Read the model definition and answer for the solid it produces. Units are mm, in the model's axes. Face numbers are marked on the shaded views. Coordinates: 2 decimals unless noted, no trailing zeros. Write each loop counter-clockwise with the first axis right and the second up, starting at its lowest first coordinate (ties: lowest second). Pieces come first, ordered by that corner, then holes. Notation, with made-up numbers: (-3.75, 78) -> (12.25, 78) arc R24 ccw to (12.25, 98) -> close; hole circle Ø6 at (60.25, 6). An arc over 180 degrees is marked (long way). One line per item, written item: value. Start each with the question number.
1. Given P1, Ø4, axis at y = -2, z = 3, coming from the +X side; P2, Ø1.9, axis at x = 0, y = 1.5, coming from the +Z side; P3, Ø6, axis at x = -3.5, z = 8, coming from the -Y side, each flat-ended and moving along its own axis, determine where each tip first touches the part or whether it passes through.
2. Consider line 1 along Y through (x, z) = (0, 8) (3 decimals); line 2 along Y through (x, z) = (0, 1.2); line 3 along Z through (x, y) = (1.25, 1). Determine where each line is inside the solid, lowest interval first.
3. Find section C-C, the plane y = -1.25. Write down the section's boundary in (x, z), and give its area (3 significant figures).
4. For a pull along X with two mould halves and no side action, classify the marked faces 1, 2, 3 and 4 as pulls with the +X half, pulls with the -X half, needs draft (parallel to the pull), parting line crosses it, or undercut.
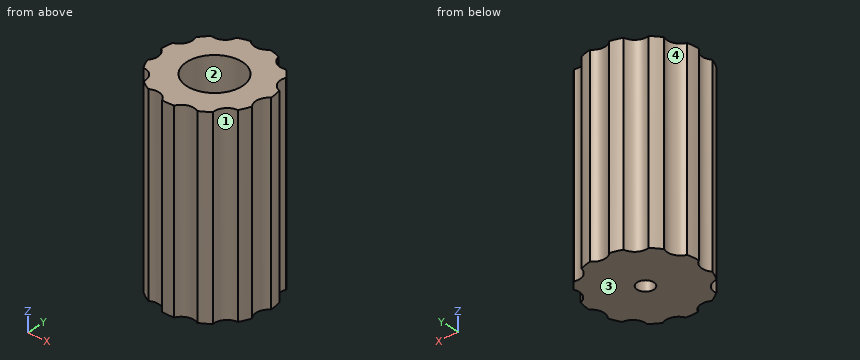
```python
from build123d import *

# Parameters (mm, degrees)
SKETCH1_R           = 6.35
BOSS_EXTRUDE1_DEPTH = 22
CUT_EXTRUDE1_DEPTH  = 23
CIRPATTERN1_COUNT   = 11
SKETCH3_R           = 3.175
CUT_EXTRUDE2_DEPTH  = 19
SKETCH4_R           = 0.9525
CUT_EXTRUDE3_DEPTH  = 4


with BuildPart() as part:
    # Sketch1 → Boss-Extrude1 (new body)
    with BuildSketch(Plane.XY):
        Circle(SKETCH1_R)
    extrude(amount=BOSS_EXTRUDE1_DEPTH)

    # Sketch2 → Cut-Extrude1 (cut, through all)
    with BuildSketch(Plane.XY.offset(22)):
        with BuildLine():
            ThreePointArc((-1.111662599, 6.251936201), (0, 5.75547169), (1.111662599, 6.251936201))
            ThreePointArc((1.111662599, 6.251936201), (0, 6.35), (-1.111662599, 6.251936201))
        make_face()
    cut_extrude1 = extrude(amount=-CUT_EXTRUDE1_DEPTH, mode=Mode.SUBTRACT)

    # CirPattern1: Cut-Extrude1 ×11 about axis
    cirpattern1_axis = Axis((0, 0, 0), (0, 0, 1))
    for i in range(1, CIRPATTERN1_COUNT):
        add(cut_extrude1.rotate(cirpattern1_axis, i * 360 / CIRPATTERN1_COUNT), mode=Mode.SUBTRACT)

    # Sketch3 → Cut-Extrude2 (cut)
    with BuildSketch(Plane.XY.offset(22)):
        Circle(SKETCH3_R)
    extrude(amount=-CUT_EXTRUDE2_DEPTH, mode=Mode.SUBTRACT)

    # Sketch4 → Cut-Extrude3 (cut, through all)
    with BuildSketch(Plane.XY.offset(3)):
        Circle(SKETCH4_R)
    extrude(amount=-CUT_EXTRUDE3_DEPTH, mode=Mode.SUBTRACT)


solid = part.part
```
Answer block:
1. P1: stops at x = 6.1
1. P2: stops at z = 3
1. P3: stops at y = -6.33
2. line 1: y = -6.35 to -3.175, 3.175 to 5.755
2. line 2: y = -6.35 to -0.95, 0.95 to 5.76
2. line 3: z = 0 to 3
3. outline: (-5.7, 0) -> (5.7, 0) -> (5.7, 22) -> (2.92, 22) -> (2.92, 3) -> (-2.92, 3) -> (-2.92, 22) -> (-5.7, 22) -> close
3. area: 140 mm2
4. face 1: pulls with the +X half
4. face 2: undercut
4. face 3: needs draft
4. face 4: pulls with the -X half
